from build123d import *

# Parameters (mm, degrees)
F0_W     = 276.38796
F0_H     = 40.325638
F0_R     = 18.45
F0_R_2   = 18.475
F0_R_3   = 18.5
F0_R_4   = 18.525
F0_R_5   = 18.55
F1_DEPTH = 4


with BuildPart() as f1:
    # F0 (on Top) → F1 (new body)
    with BuildSketch(Plane.XY):
        Rectangle(F0_W, F0_H)
        with Locations((-113.9, 0)):
            Circle(F0_R, mode=Mode.SUBTRACT)
        with Locations((-56.975, 0)):
            Circle(F0_R_2, mode=Mode.SUBTRACT)
        Circle(F0_R_3, mode=Mode.SUBTRACT)
        with Locations((57.025, 0)):
            Circle(F0_R_4, mode=Mode.SUBTRACT)
        with Locations((114.1, 0)):
            Circle(F0_R_5, mode=Mode.SUBTRACT)
    extrude(amount=F1_DEPTH)


solid = f1.part
Geometry: final body of the model. Coordinates: model frame, mm. Coordinates: 2 decimals unless noted, no trailing zeros. Loops run counter-clockwise (first coordinate to the right, second up) from the corner with the lowest first, then second, coordinate; pieces in that order, holes last. Notation, with made-up numbers: (-4.5, 81.5) - (19.5, 81.5) arc R17 cw to (19.5, 85.5) - close; hole circle Ø10 at (-23.75, 44). An arc over 180 degrees is marked (long way). One line per question, with ' | ' between items. Start each with the question number.
(1) Cut plane A-A on y = 0. Output: boundary loops of the cut face in (x, z), and give its area (3 significant figures).
(2) Draft query along X for faces 1 (the flat face through (-33, 0, 0)), 2 (the cylindrical face through (-39.353, 5.549, 1.972)), 3 (the cylindrical face through (38.518, 0.815, 1.972)). Return one class per face: +X half, -X half, draft (parallel to the pull), parting line (faces both ways), or undercut.
(3) Cut plane C-C on z = 0.95. Output: boundary loops of the cut face in (x, y) (3 decimals).
(4) Cut plane B-B on x = -113.9. Output: boundary loops of the cut face in (y, z), and give its area (3 significant figures).
(5) Cut plane D-D on x = 0. Output: boundary loops of the cut face in (y, z).
(6) Ray query, L1, parallel to X at y = 0.5, z = 3.25; L2, parallel to Y at x = 114.1, z = 3.15; L3, parallel to X at y = 2, z = 2.4. Return the intervals inside material, ascending. Write a range as from..to.
Here are the results:
1) outline: (-138.19, 0) - (-132.35, 0) - (-132.35, 4) - (-138.19, 4) - close; (-95.45, 0) - (-75.45, 0) - (-75.45, 4) - (-95.45, 4) - close; (-38.5, 0) - (-18.5, 0) - (-18.5, 4) - (-38.5, 4) - close; (18.5, 0) - (38.5, 0) - (38.5, 4) - (18.5, 4) - close; (75.55, 0) - (95.55, 0) - (95.55, 4) - (75.55, 4) - close; (132.65, 0) - (138.19, 0) - (138.19, 4) - (132.65, 4) - close | area: 366 mm²
2) face 1: draft | face 2: undercut | face 3: undercut
3) outline: (-138.194, -20.163) - (138.194, -20.163) - (138.194, 20.163) - (-138.194, 20.163) - close; hole circle Ø36.9 at (-113.9, 0); hole circle Ø36.95 at (-56.975, 0); hole circle Ø37 at (0, 0); hole circle Ø37.05 at (57.025, 0); hole circle Ø37.1 at (114.1, 0)
4) outline: (-20.16, 0) - (-18.45, 0) - (-18.45, 4) - (-20.16, 4) - close; (18.45, 0) - (20.16, 0) - (20.16, 4) - (18.45, 4) - close | area: 13.7 mm²
5) outline: (-20.16, 0) - (-18.5, 0) - (-18.5, 4) - (-20.16, 4) - close; (18.5, 0) - (20.16, 0) - (20.16, 4) - (18.5, 4) - close
6) L1: -138.19..-132.34, -95.46..-75.44, -38.51..-18.49, 18.49..38.51, 75.54..95.56, 132.64..138.19 | L2: -20.16..-18.55, 18.55..20.16 | L3: -138.19..-132.24, -95.56..-75.34, -38.61..-18.39, 18.39..38.61, 75.44..95.66, 132.54..138.19
